```python
from build123d import *

# Parameters (mm, degrees)
SKETCH1_W           = 184.15
SKETCH1_H           = 184.15
BOSS_EXTRUDE1_DEPTH = 139.7
SKETCH2_W           = 177.8
SKETCH2_H           = 177.8
CUT_EXTRUDE1_DEPTH  = 133.35
SKETCH3_R           = 5.842
BOSS_EXTRUDE2_DEPTH = 6.604


with BuildPart() as part:
    # Sketch1 → Boss-Extrude1 (new body)
    with BuildSketch(Plane(origin=(0, 0, 0), x_dir=(1, 0, 0), z_dir=(0, 1, 0))):
        Rectangle(SKETCH1_W, SKETCH1_H)
    extrude(amount=BOSS_EXTRUDE1_DEPTH)

    # Sketch2 → Cut-Extrude1 (cut)
    with BuildSketch(Plane(origin=(0, 139.7, 0), x_dir=(1, 0, 0), z_dir=(0, 1, 0))):
        Rectangle(SKETCH2_W, SKETCH2_H)
    extrude(amount=-CUT_EXTRUDE1_DEPTH, mode=Mode.SUBTRACT)

    # Sketch3 → Boss-Extrude2 (add)
    with BuildSketch(Plane(origin=(0, 6.35, 0), x_dir=(1, 0, 0), z_dir=(0, 1, 0))):
        with Locations((-1.016, 78.651394374)):
            Circle(SKETCH3_R)
    extrude(amount=BOSS_EXTRUDE2_DEPTH)


solid = part.part
```
Could you check a few things on this model? Use its own coordinates, in mm. A direction names the side the tool comes from. Coordinates: 2 decimals unless noted, no trailing zeros. Write each loop counter-clockwise with the first axis right and the second up, starting at its lowest first coordinate (ties: lowest second). Pieces come first, ordered by that corner, then holes. Notation, with made-up numbers: M -2.5,69.25 L 7.5,69.25 A8 cw 7.5,74.25 Z; hole C 49,17 d11. An arc over 180 degrees is marked long. Answer as CSV lines item,"result". Start each with the question number.
1) I want a section at B-B, the plane z = -7.5. Please give me the cut outline in (x, y) (3 decimals), and give its area (3 significant figures).
2) I want a section at A-A, the plane y = 65. Please give me the cut outline in (x, z) (3 decimals).
3) Please list where these lines run through material, in increasing order: line 1 (Z direction, x = -51, y = 32.5) (3 decimals); line 2 (Y direction, x = 57.5, z = -37). Write a range as from..to.
4) We'd pull the mould along Z, two halves only. Please class faces 3 (the cylindrical face through (-1.777, 9.606, -84.444)), 4 (the flat face through (-1, 0, -1)), 5 (the flat face through (-1, 74, -88.9)), 6 (the flat face through (-1, 69, -92.075)): +Z half, -Z half, draft (parallel to the pull), parting line (faces both ways), or undercut.
5) I want a section at C-C, the plane x = 55. Please give me the cut outline in (y, z) (3 decimals), and give its area (3 significant figures).
6) For faces 1 (the flat face through (88.9, 74, 1)), 2 (the flat face through (92.075, 69, 1)), which set-ups out of +Z, -Z, +X, -X, +Y, -Y let a thin tool reach every point of the face, with its end or its side?
7) For P1, Ø13, axis at x = -4, z = -77, coming from the +Y side; P2, Ø10, axis at x = 71, z = 0, coming from the -Y side; P3, Ø3, axis at x = -45, z = -12.5, coming from the +Y side, each with a flat end and sliding along its axis, tell me the tip position at first contact or that it passes through.
Data:
1,outline,"M -92.075,0 L 92.075,0 L 92.075,139.7 L 88.9,139.7 L 88.9,6.35 L -88.9,6.35 L -88.9,139.7 L -92.075,139.7 Z"
1,area,"2,020 mm^2"
2,outline,"M -92.075,-92.075 L 92.075,-92.075 L 92.075,92.075 L -92.075,92.075 Z; hole M -88.9,-88.9 L 88.9,-88.9 L 88.9,88.9 L -88.9,88.9 Z"
3,line 1,"z = -92.075..-88.9, 88.9..92.075"
3,line 2,"y = 0..6.35"
4,face 3,"undercut"
4,face 4,"draft"
4,face 5,"undercut"
4,face 6,"-Z half"
5,outline,"M 0,-92.075 L 139.7,-92.075 L 139.7,-88.9 L 6.35,-88.9 L 6.35,88.9 L 139.7,88.9 L 139.7,92.075 L 0,92.075 Z"
5,area,"2,020 mm^2"
6,face 1,"+Y"
6,face 2,"+Z, -Z, +X, +Y, -Y"
7,P1,"stops at y = 12.95"
7,P2,"stops at y = 0"
7,P3,"stops at y = 6.35"
